Check sheet for the drawn part. Datum: minimum x, y, z corner. Units: mm. Round coordinates to 2 decimals unless told otherwise and drop trailing zeros. Write each loop counter-clockwise with the first axis right and the second up, starting at its lowest first coordinate (ties: lowest second). Pieces come first, ordered by that corner, then holes. Notation, with made-up numbers: M 68.25,-35.5 L 93.25,-35.5 A12 cw 93.25,-18.5 Z; hole C 78.5,57.25 d6. An arc over 180 degrees is marked long. Use a Markdown table: item, result.
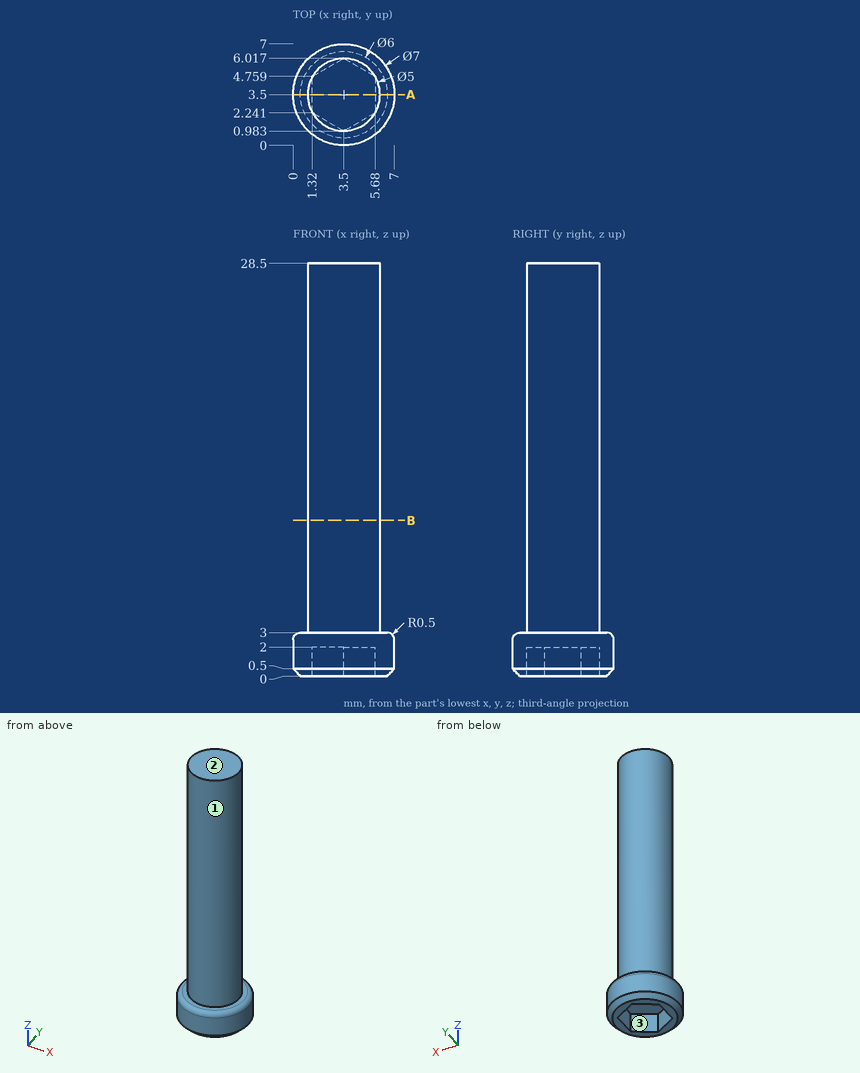
Item 1: Cross-section at A-A, the plane y = 3.5. Record the cut outline in (x, z), and give its area (3 significant figures).
Outcome:
| item | result |
|---|---|
| outline | M 0,0.5 L 0.5,0 L 1.32,0 L 1.32,2 L 5.68,2 L 5.68,0 L 6.5,0 L 7,0.5 L 7,2.5 A0.5 ccw 6.5,3 L 6,3 L 6,28.5 L 1,28.5 L 1,3 L 0.5,3 A0.5 ccw 0,2.5 Z |
| area | 139 mm2 |
Item 2: Cross-section at B-B, the plane z = 10.75. Record the cut outline in (x, y), and give its area (3 significant figures).
Outcome:
| item | result |
|---|---|
| outline | C 3.5,3.5 d5 |
| area | 19.6 mm2 |
Item 3: Material ranges on line 1 along Z through (x, y) = (2, 2.25); line 2 along Z through (x, y) = (6, 4.5); line 3 along X through (y, z) = (3.75, 15.5), recorded low to high. Write a range as from..to.
Outcome:
| item | result |
|---|---|
| line 1 | z = 2..28.5 |
| line 2 | z = 0..3 |
| line 3 | x = 1.01..5.99 |
Item 4: Go/stop test with flat-tipped pins: pin 1 (3 mm diameter, centred on x = 6.5, y = 4, fed in from +Z); pin 2 (1.5 mm diameter, centred on y = 5, z = 16.5, fed in from +X) (1 decimal); pin 3 (1.5 mm diameter, centred on y = 5, z = 4, fed in from -X) (1 decimal); pin 4 (2 mm diameter, centred on x = 3.5, y = 2.5, fed in from -Z). Record where each tip stops, or that it passes through.
Outcome:
| item | result |
|---|---|
| pin 1 | stops at z = 28.5 |
| pin 2 | stops at x = 5.9 |
| pin 3 | stops at x = 1.1 |
| pin 4 | stops at z = 2 |
Item 5: Mould release check, pull along X, two halves, no side actions. Record for the marked faces 1, 2 and 3: +X half, -X half, draft (parallel to the pull), parting line (faces both ways), or undercut.
Outcome:
| item | result |
|---|---|
| face 1 | parting line |
| face 2 | draft |
| face 3 | undercut |
